For this review, take the finished solid that the model builds, in its own axes (mm). A direction names the side the tool comes from. Round coordinates to 2 decimals unless told otherwise and drop trailing zeros. Order: outer loops, then holes, each group sorted by start corner. A loop starts at its lowest first (then second) coordinate and runs counter-clockwise, first axis right, second up. Notation, with made-up numbers: M 82.25,-10.5 L 131.25,-10.5 A15 cw 131.25,8.5 Z; hole C 59.5,-9.75 d9. An arc over 180 degrees is marked long. Answer in a Markdown table with one row per item. Add a question column.
```python
from build123d import *

# Parameters (mm, degrees)
SKETCH1_W                = 68
SKETCH1_H                = 18
BOSS_EXTRUDE1_DEPTH      = 46
BOSS_EXTRUDE2_DEPTH      = 40
FILLET1_R                = 12
FILLET3_R                = 18
FILLET4_R                = 12
BOSS_EXTRUDE3_DEPTH      = 37
BOSS_EXTRUDE3_DEPTH_BACK = 18
SKETCH3_R                = 40
HOLE1_D                  = 40
BOSS_EXTRUDE5_DEPTH      = 7
FILLET5_R                = 12
HOLE2_D                  = 10


with BuildPart() as part:
    # Sketch1 → Boss-Extrude1 (new, symmetric)
    with BuildSketch(Plane(origin=(0, 0, 0), x_dir=(0, 0, -1), z_dir=(1, 0, 0))):
        Rectangle(SKETCH1_W, SKETCH1_H)
    extrude(amount=BOSS_EXTRUDE1_DEPTH, both=True)

    # Sketch2 → Boss-Extrude2 (add, symmetric)
    with BuildSketch(Plane(origin=(0, 0, 0), x_dir=(0, 0, -1), z_dir=(1, 0, 0))):
        Polygon((34, 9), (22, 9), (22, 111), (91, 111), (91, 99), (34, 99), align=None)
    extrude(amount=BOSS_EXTRUDE2_DEPTH, both=True)

    # Fillet1
    # the kernel refuses this fillet: 12 mm, written as the material it adds along each edge
    with BuildSketch(Plane(origin=(-40, 9, -34), x_dir=(-1, 0, 0), z_dir=(0, 0, 1))) as fillet1_piece_1:
        with BuildLine():
            CenterArc((12, -10.392304845), FILLET1_R, 120, 60)
            Line((0, -10.392304845), (-0.24, -10.392304845))
            Line((-0.24, -10.392304845), (-0.24, 0))
            Line((-0.24, 0), (0, 0.24))
            ThreePointArc((0, 0.24), (3, 0.24), (5.88, 0.207846097))
            Line((5.88, 0.207846097), (6, 0))
        make_face()
    extrude(amount=12)
    with BuildSketch(Plane(origin=(40, 9, -34), x_dir=(1, 0, 0), z_dir=(0, 0, 1))) as fillet1_piece_2:
        with BuildLine():
            CenterArc((12, 10.392304845), FILLET1_R, 180, 60)
            Line((0, 10.392304845), (-0.24, 10.392304845))
            Line((-0.24, 10.392304845), (-0.24, 0))
            Line((-0.24, 0), (0, -0.24))
            ThreePointArc((0, -0.24), (3, -0.24), (5.88, -0.207846097))
            Line((5.88, -0.207846097), (6, 0))
        make_face()
    extrude(amount=12)

    # Fillet3
    fillet3_edges = [part.edges().sort_by_distance(p)[0] for p in [
        (0, 111, -22),
    ]]
    fillet(fillet3_edges, radius=FILLET3_R)

    # Fillet4
    fillet4_edges = [part.edges().sort_by_distance(p)[0] for p in [
        (0, 99, -34),
    ]]
    fillet(fillet4_edges, radius=FILLET4_R)

    # Sketch3 → Boss-Extrude3 (add, two sides: drawn at the far end of the back side and taken through both)
    with BuildSketch(Plane(origin=(0, 111, 0), x_dir=(1, 0, 0), z_dir=(0, 1, 0)).offset(-BOSS_EXTRUDE3_DEPTH_BACK)):
        with Locations(Location((0, 91, 0), (0, 0, 270))):
            Circle(SKETCH3_R)
    extrude(amount=BOSS_EXTRUDE3_DEPTH + BOSS_EXTRUDE3_DEPTH_BACK)

    # Hole1 (through all)
    with Locations(Plane(origin=(0, 148, 0), x_dir=(1, 0, 0), z_dir=(0, 1, 0))):
        with Locations((0, 91)):
            Hole(HOLE1_D / 2)

    # Sketch6 → Boss-Extrude5 (add, symmetric)
    with BuildSketch(Plane(origin=(0, 0, 0), x_dir=(0, 0, -1), z_dir=(1, 0, 0))):
        with BuildLine():
            Line((-34, 9), (-19.470663618, 99.647109079))
            ThreePointArc((-19.470663618, 99.647109079), (-5.682290367, 124.586243842), (20.849974888, 134.984252313))
            Line((20.849974888, 134.984252313), (57.932127912, 136))
            Line((57.932127912, 136), (57.932127912, 111))
            Line((57.932127912, 111), (40, 111))
            ThreePointArc((40, 111), (27.272077939, 105.727922061), (22, 93))
            Line((22, 93), (22, 19.392304845))
            Line((22, 19.392304845), (22, 9))
            Line((22, 9), (-34, 9))
        make_face()
    extrude(amount=BOSS_EXTRUDE5_DEPTH, both=True)

    # Fillet5
    fillet5_edges = [part.edges().sort_by_distance(p)[0] for p in [
        (3.513591356, 135.814351592, -51.154615377),
    ]]
    fillet(fillet5_edges, radius=FILLET5_R)

    # Hole2 (through all)
    with Locations(Plane(origin=(0, 9, 0), x_dir=(1, 0, 0), z_dir=(0, 1, 0))):
        with Locations((26, -6)):
            hole2 = Hole(HOLE2_D / 2)

    # Mirror1: Hole2 across plane
    add(hole2.mirror(Plane(origin=(0, 0, 0), x_dir=(0, 0, 1), z_dir=(1, 0, 0))), mode=Mode.SUBTRACT)


solid = part.part
```
1. Consider section D-D on y = 39. Write out the cut boundary in (x, z).
2. Consider section C-C on x = 26. Write out the cut boundary in (y, z).
3. Clearance check with flat-ended pins moving along their axes: pin 1 Ø12 at (x, z) = (-3, -57.5) entering from -Y; pin 2 Ø10 at (x, y) = (-31, 110.5) entering from -Z; pin 3 Ø5 at (x, z) = (-3, -109) entering from +Y; pin 4 Ø1 at (x, y) = (19, 75.5) entering from +Z. State where each tip first meets the part, or that it passes through.
4. The part is to be moulded in two halves that separate along X. For faces 5 (the flat face through (27, 9, 13)), 6 (the flat face through (-46, 0, 0)), 7 (the cylindrical face through (-31, 0, 6)), say which applies: pulls with the +X half, pulls with the -X half, needs draft (parallel to the pull), parting line crosses it, or undercut.
5. Consider section A-A on z = 6. Write out the cut boundary in (x, y).
6. Consider section B-B on y = 4. Write out the cut boundary in (x, z).
7. To check wall thickness, follow probe 1 along Z at (x, y) = (-26, -1); probe 2 along X at (y, z) = (125, -91); probe 3 along Z at (x, y) = (-37.5, 70). State the ranges of each line that lie inside material, in increasing order. Write a range as [from, to].
8. For faces 1 (the flat face through (40, 79, -33.7)), 2 (the flat face through (1, 40, -34)), 3 (the flat face through (27, 111, -54)), 4 (the flat face through (3, 99, -50)), list the 3-axis set-ups (+Z, -Z, +X, -X, +Y, -Y) from which the entire face can be reached by the end or side of a thin tool; tool diameter is ignored.
Solved:
| question | item | result |
|---|---|---|
| 1 | outline | M -40,-34 L 40,-34 L 40,-22 L 7,-22 L 7,29.19 L -7,29.19 L -7,-22 L -40,-22 Z |
| 2 | outline | M -9,-34 L 87,-34 A12 cw 99,-46 L 99,-60.6 L 93,-60.6 L 93,-121.4 L 148,-121.4 L 148,-60.6 L 111,-60.6 L 111,-40 A18 ccw 93,-22 L 9,-22 L 9,1 L -9,1 Z; M -9,11 L 9,11 L 9,34 L -9,34 Z |
| 3 | pin 1 | stops at y = 93 |
| 3 | pin 2 | stops at z = -121.4 |
| 3 | pin 3 | stops at y = 148 |
| 3 | pin 4 | stops at z = -22 |
| 4 | face 5 | needs draft |
| 4 | face 6 | pulls with the -X half |
| 4 | face 7 | undercut |
| 5 | outline | M -46,-9 L -31,-9 L -31,9 L -46,9 Z; M -21,-9 L 21,-9 L 21,9 L 7,9 L 7,124.3 L -7,124.3 L -7,9 L -21,9 Z; M 31,-9 L 46,-9 L 46,9 L 31,9 Z |
| 6 | outline | M -46,-34 L 46,-34 L 46,34 L -46,34 Z; hole C -26,6 d10; hole C 26,6 d10 |
| 7 | probe 1 | z = [-34, 1], [11, 34] |
| 7 | probe 2 | x = [-40, -20], [20, 40] |
| 7 | probe 3 | z = [-34, -22] |
| 8 | face 1 | +Z, -Z, +X, +Y |
| 8 | face 2 | -Z, +X, -X, -Y |
| 8 | face 3 | +Z, +X, +Y |
| 8 | face 4 | -Y |
